Design review of the part built by this model. Coordinates are the model's own, in mm. A direction names the side the tool comes from. Coordinates: 2 decimals unless noted, no trailing zeros. Loops run counter-clockwise (first coordinate to the right, second up) from the corner with the lowest first, then second, coordinate; pieces in that order, holes last. Notation, with made-up numbers: (10.25, -13) -> (48.25, -13) arc R16 ccw to (48.25, 9) -> close; hole circle Ø4 at (62.25, 88). An arc over 180 degrees is marked (long way). Use one line per item in the form item = value. Start each with the question number.
1. Machinability: for faces 4 (the face through (51.181, 30, 10)), 5 (the face through (27, 31, 23.495)), 6 (the face through (18, 65, 5.08)), which of the approach directions +Z, -Z, +X, -X, +Y, -Y give a long, thin tool a straight path to every point of the face, cutting with its end or side? Answer none if there is none.
2. Consider section D-D (x = 14). State the section outline as (y, z) points (1 decimal), then the cut area to 3 significant figures.
3. Consider section C-C (x = 35.5). State the section outline as (y, z) points (3 decimals).
4. Consider section B-B (y = 12). State the section outline as (x, z) points (3 decimals), then the cut area to 3 significant figures.
5. Wall thickness on line 1 (Y direction, x = 11, z = 10); line 2 (X direction, y = 40, z = 12.5); line 3 (Z direction, x = 36, y = 8.5) (3 decimals): over which ranges is each line inside the solid? List them lowest first. Write a range as from..to.
6. The part is to be moulded in two halves that separate along Y. For faces 1 (the face through (28, 60.198, 12)), 2 (the face through (18, -4, 5.08)), 3 (the face through (4.193, 4.153, 9.893)), say which applies: released by +Y, released by -Y, zero draft, split by the parting line, or undercut.
7. Consider section A-A (z = 14.5). State the section outline as (x, y) points, then the cut area to 3 significant figures.
8. For pin 1 (7 mm diameter, centred on x = 22.5, z = 6.5, fed in from +Y); pin 2 (4.5 mm diameter, centred on x = 17.68, y = -7.57, fed in from +Z); pin 3 (7.5 mm diameter, centred on x = 13.5, y = -4.5, fed in from +Z); pin 4 (6 mm diameter, centred on x = 28.5, z = 12.5, fed in from -Y), all flat-tipped, find the tip position at first contact; note any pin that passes through.
from build123d import *

# Parameters (mm, degrees)
BOSS_EXTRUDE1_DEPTH = 23.495
SHELL1_T            = -3.429
FILLET1_R           = 2.54
SKETCH2_R           = 7.5692
SKETCH2_R_2         = 2.4892
BOSS_EXTRUDE2_DEPTH = 5.08
CUT_EXTRUDE1_REACH  = 56.61
SKETCH3_W           = 3.81
SKETCH3_H           = 40.3352
FILLET2_R           = 1.27


with BuildPart() as part:
    # Sketch1 → Boss-Extrude1 (new body)
    with BuildSketch(Plane.XY):
        with BuildLine():
            Line((2.54, 0), (52.07, 0))
            ThreePointArc((52.07, 0), (53.866051224, 0.743948776), (54.61, 2.54))
            Line((54.61, 2.54), (54.61, 57.658))
            ThreePointArc((54.61, 57.658), (53.866051224, 59.454051224), (52.07, 60.198))
            Line((52.07, 60.198), (2.54, 60.198))
            ThreePointArc((2.54, 60.198), (0.743948776, 59.454051224), (0, 57.658))
            Line((0, 57.658), (0, 2.54))
            ThreePointArc((0, 2.54), (0.743948776, 0.743948776), (2.54, 0))
        make_face()
    extrude(amount=BOSS_EXTRUDE1_DEPTH)

    # Shell1
    shell1_openings = [part.faces().sort_by_distance(p)[0] for p in [
        (27.305, 30.099, 0),
    ]]
    offset(amount=SHELL1_T, openings=shell1_openings, kind=Kind.INTERSECTION)

    # Fillet1
    fillet1_edges = [part.edges().sort_by_distance(p)[0] for p in [
        (3.429, 3.429, 10.033),
        (51.181, 3.429, 10.033),
        (51.181, 56.769, 10.033),
        (3.429, 56.769, 10.033),
    ]]
    fillet(fillet1_edges, radius=FILLET1_R)

    # Sketch2 → Boss-Extrude2 (add)
    with BuildSketch(Plane(origin=(0, 0, 0), x_dir=(-1, 0, 0), z_dir=(0, 0, -1))):
        with BuildLine():
            ThreePointArc((-17.6784, 60.198), (-23.030632648, 62.414967352), (-25.2476, 67.7672))
            ThreePointArc((-25.2476, 67.7672), (-27.464567352, 62.414967352), (-32.8168, 60.198))
            Line((-32.8168, 60.198), (-17.6784, 60.198))
        make_face()
        with Locations((-17.6784, 67.7672)):
            Circle(SKETCH2_R)
        with Locations((-17.6784, 67.7672)):
            Circle(SKETCH2_R_2, mode=Mode.SUBTRACT)
        with BuildLine():
            ThreePointArc((-2.54, 60.198), (-7.892232648, 62.414967352), (-10.1092, 67.7672))
            ThreePointArc((-10.1092, 67.7672), (-12.326167352, 62.414967352), (-17.6784, 60.198))
            Line((-17.6784, 60.198), (-2.54, 60.198))
        make_face()
        with Locations((-17.6784, -7.5692)):
            Circle(SKETCH2_R)
        with Locations((-17.6784, -7.5692)):
            Circle(SKETCH2_R_2, mode=Mode.SUBTRACT)
        with BuildLine():
            ThreePointArc((-32.8168, 0), (-27.464567352, -2.216967352), (-25.2476, -7.5692))
            ThreePointArc((-25.2476, -7.5692), (-23.03063266, -2.216967364), (-17.678400033, 0))
            Line((-17.678400033, 0), (-32.8168, 0))
        make_face()
        with BuildLine():
            ThreePointArc((-17.678400033, 0), (-12.326167364, -2.21696734), (-10.1092, -7.5692))
            ThreePointArc((-10.1092, -7.5692), (-7.892232648, -2.216967352), (-2.54, 0))
            Line((-2.54, 0), (-17.678400033, 0))
        make_face()
    extrude(amount=-BOSS_EXTRUDE2_DEPTH)

    # Sketch3 → Cut-Extrude1 (cut, up to next)
    with BuildSketch(Plane.ZY, mode=Mode.PRIVATE) as cut_extrude1_sk1:
        with Locations((1.905, 26.1366)):
            Rectangle(SKETCH3_W, SKETCH3_H)
    cut_extrude1_tool1 = extrude(cut_extrude1_sk1.sketch, amount=-CUT_EXTRUDE1_REACH, mode=Mode.PRIVATE) & part.part
    add(cut_extrude1_tool1.solids().sort_by_distance((0, 26.1366, 1.905))[0], mode=Mode.SUBTRACT)

    # Fillet2
    fillet2_edges = [part.edges().sort_by_distance(p)[0] for p in [
        (3.429, 46.3042, 1.905),
        (3.429, 5.969, 1.905),
        (0, 5.969, 1.905),
        (0, 46.3042, 1.905),
    ]]
    fillet(fillet2_edges, radius=FILLET2_R)


solid = part.part
Geometry check:
q1.face_4 = -Z
q1.face_5 = +Z, +X, -X, +Y, -Y
q1.face_6 = +Z, +X, -X, +Y
q2.outline = (-14.2, 0) -> (3.4, 0) -> (3.4, 20.1) -> (56.8, 20.1) -> (56.8, 0) -> (74.4, 0) -> (74.4, 5.1) -> (60.2, 5.1) -> (60.2, 23.5) -> (0, 23.5) -> (0, 5.1) -> (-14.2, 5.1) -> close
q2.area = 488 mm²
q3.outline = (0, 0) -> (3.429, 0) -> (3.429, 20.066) -> (56.769, 20.066) -> (56.769, 0) -> (60.198, 0) -> (60.198, 23.495) -> (0, 23.495) -> close
q4.outline = (0, 3.81) -> (3.429, 3.81) -> (3.429, 20.066) -> (51.181, 20.066) -> (51.181, 0) -> (54.61, 0) -> (54.61, 23.495) -> (0, 23.495) -> close
q4.area = 312 mm²
q5.line_1 = 0..3.43, 56.77..60.2
q5.line_2 = 0..3.43, 51.18..54.61
q5.line_3 = 20.066..23.495
q6.face_1 = released by +Y
q6.face_2 = zero draft
q6.face_3 = undercut
q7.outline = (0, 2.54) arc R2.54 ccw to (2.54, 0) -> (52.07, 0) arc R2.54 ccw to (54.61, 2.54) -> (54.61, 57.66) arc R2.54 ccw to (52.07, 60.2) -> (2.54, 60.2) arc R2.54 ccw to (0, 57.66) -> close; hole (3.43, 5.97) arc R2.54 ccw to (5.97, 3.43) -> (48.64, 3.43) arc R2.54 ccw to (51.18, 5.97) -> (51.18, 54.23) arc R2.54 ccw to (48.64, 56.77) -> (5.97, 56.77) arc R2.54 ccw to (3.43, 54.23) -> close
q7.area = 740 mm²
q8.pin_1 = 75.16
q8.pin_2 = through
q8.pin_3 = 5.08
q8.pin_4 = 0
